from build123d import *

# Parameters (mm, degrees)
SKETCH1_R           = 254
BOSS_EXTRUDE1_DEPTH = 635


with BuildPart() as part:
    # Sketch1 → Boss-Extrude1 (new body)
    with BuildSketch(Plane(origin=(0, 0, 0), x_dir=(1, 0, 0), z_dir=(0, 1, 0))):
        with BuildLine():
            Line((0, -508), (0, 508))
            Line((0, 508), (508, 508))
            Line((508, 508), (508, 254))
            Line((508, 254), (762, 254))
            Line((762, 254), (762, 508))
            Line((762, 508), (1752.6, 508))
            ThreePointArc((1752.6, 508), (2260.6, 0), (1752.6, -508))
            Line((1752.6, -508), (762, -508))
            Line((762, -508), (762, -254))
            Line((762, -254), (508, -254))
            Line((508, -254), (508, -508))
            Line((508, -508), (0, -508))
        make_face()
        with Locations(Location((1752.6, 0, 0), (0, 0, 90))):
            Circle(SKETCH1_R, mode=Mode.SUBTRACT)
    extrude(amount=BOSS_EXTRUDE1_DEPTH)


solid = part.part
Verification items for the finished model (mm, model axes). A direction names the side the tool comes from. Coordinates: 2 decimals unless noted, no trailing zeros. Order: outer loops, then holes, each group sorted by start corner. A loop starts at its lowest first (then second) coordinate and runs counter-clockwise, first axis right, second up. Notation, with made-up numbers: M 29.25,46 L 43.25,46 A18 cw 43.25,59 Z; hole C 79.5,12 d3. An arc over 180 degrees is marked long. One line per item, written item: value. Start each with the question number.
Item 1: Sectioned sample at C-C on x = 1615. Record the cut outline in (y, z), then the cut area to 3 significant figures.
Item 2: Depth check by flat-ended pin: P1, Ø3, axis at x = 868, z = -91, coming from the -Y side; P2, Ø4, axis at y = 514, z = -349.5, coming from the +X side; P3, Ø10, axis at y = 315.5, z = -212, coming from the +X side; P4, Ø8, axis at y = 384.5, z = 368, coming from the +X side. Enter the tip coordinate at first touch or a pass-through.
Item 3: Access from +Z, -Z, +X, -X, +Y, -Y to the whole of each face (thin tool, end or side, straight path). Record for faces 4 (the flat face through (637, 313, 254)), 5 (the flat face through (250, 313, -508)), 6 (the flat face through (762, 313, -379)).
Item 4: Sectioned sample at B-B on y = 565. Record the cut outline in (x, z), then the cut area to 3 significant figures.
Item 5: Sectioned sample at A-A on z = 0. Record the cut outline in (x, y), then the cut area to 3 significant figures.
Item 6: Mould release check, pull along X, two halves, no side actions. Record for faces 1 (the flat face through (1146, 635, -7)), 2 (the flat face through (0, 313, 7)), 3 (the flat face through (762, 313, 383)): pulls with the +X half, pulls with the -X half, needs draft (parallel to the pull), parting line crosses it, or undercut.
Item 7: Thickness scan on probe 1 along X at (y, z) = (170, 0); probe 2 along Z at (x, y) = (1752.6, 453); probe 3 along X at (y, z) = (56, 192). Record the ranges inside material, lowest first.
Calculated:
1. outline: M 0,-508 L 635,-508 L 635,-213.5 L 0,-213.5 Z; M 0,213.5 L 635,213.5 L 635,508 L 0,508 Z
1. area: 374,000 mm^2
2. P1: y = 0
2. P2: x = 2123.15
2. P3: x = 2216.51
2. P4: x = 2106.96
3. face 4: +Z, +Y, -Y
3. face 5: -Z, +X, -X, +Y, -Y
3. face 6: -Z, +Y, -Y
4. outline: M 0,-508 L 508,-508 L 508,-254 L 762,-254 L 762,-508 L 1752.6,-508 A508 ccw 1752.6,508 L 762,508 L 762,254 L 508,254 L 508,508 L 0,508 Z; hole C 1752.6,0 d508
4. area: 1,850,000 mm^2
5. outline: M 0,0 L 1498.6,0 L 1498.6,635 L 0,635 Z; M 2006.6,0 L 2260.6,0 L 2260.6,635 L 2006.6,635 Z
5. area: 1,110,000 mm^2
6. face 1: needs draft
6. face 2: pulls with the -X half
6. face 3: undercut
7. probe 1: 0 to 1498.6, 2006.6 to 2260.6
7. probe 2: -508 to -254, 254 to 508
7. probe 3: 0 to 1586.31, 1918.89 to 2222.92
